```python
from build123d import *
from build123d.topology import SkipClean

# Parameters (mm, degrees)
SKETCH_1_W      = 47
SKETCH_1_H      = 38
SKETCH_1_R      = 1.5
EXTRUDE_1_DEPTH = 3
SKETCH_2_W      = 47
SKETCH_2_H      = 11
SKETCH_2_R      = 1.5
EXTRUDE_2_DEPTH = 7
EXTRUDE_3_DEPTH = 8
FILLET_4_R      = 3
EXTRUDE_4_DEPTH = 10
FILLET_6_R      = 3
EXTRUDE_START   = 3
SKETCH_7_R      = 3.5
SKETCH_7_R_2    = 1.5
EXTRUDE_5_DEPTH = 3


with BuildPart() as part:
    # 草图1 → 凸台-拉伸1 (new body)
    with BuildSketch(Plane(origin=(0, 0, 0), x_dir=(1, 0, 0), z_dir=(0, 1, 0))):
        Rectangle(SKETCH_1_W, SKETCH_1_H)
        with Locations(Location((19.5, 14, 0), (0, 0, 270))):
            Circle(SKETCH_1_R, mode=Mode.SUBTRACT)
        with Locations(Location((19.5, -14, 0), (0, 0, 270))):
            Circle(SKETCH_1_R, mode=Mode.SUBTRACT)
        with Locations(Location((-19.5, -14, 0), (0, 0, 270))):
            Circle(SKETCH_1_R, mode=Mode.SUBTRACT)
        with Locations(Location((-19.5, 14, 0), (0, 0, 270))):
            Circle(SKETCH_1_R, mode=Mode.SUBTRACT)
    extrude(amount=EXTRUDE_1_DEPTH)

    # 草图2 → 凸台-拉伸2 (add)
    with BuildSketch(Plane.XY.offset(19)):
        with Locations((0, 5.5)):
            Rectangle(SKETCH_2_W, SKETCH_2_H)
        with Locations((-17.5, 7)):
            Circle(SKETCH_2_R, mode=Mode.SUBTRACT)
        with Locations((-9.5, 7)):
            Circle(SKETCH_2_R, mode=Mode.SUBTRACT)
    extrude(amount=EXTRUDE_2_DEPTH)

    # 草图3 → 凸台-拉伸3 (add)
    with BuildSketch(Plane(origin=(0, 0, 0), x_dir=(0, 0, -1), z_dir=(1, 0, 0))):
        Polygon((-19, 11), (-19, 8), (-4, 3), (5, 3), align=None)
    extrude(amount=EXTRUDE_3_DEPTH)

    # 圆角4
    fillet_4_edges = [part.edges().sort_by_distance(p)[0] for p in [
        (-23.5, 11, 22.5),
        (23.5, 11, 22.5),
    ]]
    fillet(fillet_4_edges, radius=FILLET_4_R)

    # 草图4 → 凸台-拉伸4 (add)
    with BuildSketch(Plane.ZY.offset(23.5)):
        Polygon((26, 0), (26, -5), (23, -5), (19.5, 0), align=None)
    extrude_4 = extrude(amount=-EXTRUDE_4_DEPTH)

    # 镜向1: 凸台-拉伸4 across plane
    add(extrude_4.mirror(Plane(origin=(0, 0, 0), x_dir=(0, 0, 1), z_dir=(1, 0, 0))))

    # 圆角6
    fillet_6_edges = [part.edges().sort_by_distance(p)[0] for p in [
        (-23.5, 1.5, -19),
        (23.5, 1.5, -19),
    ]]
    fillet(fillet_6_edges, radius=FILLET_6_R)

    # 草图7 → 凸台-拉伸5 (add)
    with SkipClean():  # the faces are left unmerged after this step: merging them gives an invalid solid
        with BuildSketch(Plane(origin=(0, 0, 19), x_dir=(-1, 0, 0), z_dir=(0, 0, -1)).offset(EXTRUDE_START)):
            with Locations(Location((9.5, 7, 0), (0, 0, 180))):
                Circle(SKETCH_7_R)
            with Locations((9.5, 7)):
                Circle(SKETCH_7_R_2, mode=Mode.SUBTRACT)
        extrude(amount=-EXTRUDE_5_DEPTH)


solid = part.part
```
Source: CAD feature listing. Evaluate the final solid. Frame: model axes, mm. A direction names the side the tool comes from. Give positions to 0.01 mm unless a question says otherwise; leave off trailing zeros. Write each loop counter-clockwise with the first axis right and the second up, starting at its lowest first coordinate (ties: lowest second). Pieces come first, ordered by that corner, then holes. Notation, with made-up numbers: (-37.5, 55) - (-15.5, 55) arc R19 cw to (-15.5, 78) - close; hole circle Ø7 at (11.5, 83). An arc over 180 degrees is marked (long way). One line per item, written item: value. Start each with the question number.
Q1. Set-up query: faces 1 (the face through (-13.5, -2, 24)), 2 (the face through (-12.3, 9.1, 17.5)), 3 (the face through (0, 6, 10)). Return all of +Z, -Z, +X, -X, +Y, -Y with unobstructed straight access to the full face (end or side cutting, diameter ignored); none if empty.
Q2. First-contact query: pin 1 Ø13.5 at (x, z) = (-1, 5.5) entering from -Y; pin 2 Ø3.5 at (x, y) = (-9.5, 7) entering from +Z; pin 3 Ø5 at (x, z) = (-19.5, 14) entering from +Y; pin 4 Ø4 at (x, z) = (3.5, 13) entering from +Y. Flat tips, straight axial feed; report the tip coordinate or a pass-through.
Q3. Section query D-D, the plane x = 19.5. Return the cut outline in (y, z), then the cut area to 3 significant figures.
Q4. Material intervals for probe 1 along X at (y, z) = (1.5, -14); probe 2 along Y at (x, z) = (-9, -9.5); probe 3 along Z at (x, y) = (-19, 0.25), sorted ascending. Write a range as from..to.
Q5. Section query A-A, the plane z = -14. Return the cut outline in (x, y), then the cut area to 3 significant figures.
Q6. Draft query along Z for faces 4 (the face through (-19, -5, 25)), 5 (the face through (20.51, 1.48, 12.89)), 6 (the face through (0, 1, -19)). Return one class per face: +Z half, -Z half, draft (parallel to the pull), parting line (faces both ways), or undercut.
Answer:
1. face 1: +Z, -Z, -Y
1. face 2: -Z
1. face 3: -Z, +Y
2. pin 1: stops at y = 0
2. pin 2: stops at z = 26
2. pin 3: stops at y = 3
2. pin 4: stops at y = 9.67
3. outline: (-5, 23) - (0, 19.5) - (0, 15.5) - (3, 15.5) - (3, 19) - (11, 19) - (11, 26) - (-5, 26) - close; (0, -19) - (3, -19) - (3, -15.5) - (0, -15.5) - close; (0, -12.5) - (3, -12.5) - (3, 12.5) - (0, 12.5) - close
3. area: 197 mm2
4. probe 1: x = -23.5..-21, -18..18, 21..23.5
4. probe 2: y = 0..3
4. probe 3: z = -19..-15.41, -12.59..12.59, 15.41..26
5. outline: (-23.5, 0) - (-21, 0) - (-21, 3) - (-23.5, 3) - close; (-18, 0) - (18, 0) - (18, 3) - (-18, 3) - close; (21, 0) - (23.5, 0) - (23.5, 3) - (21, 3) - close
5. area: 123 mm2
6. face 4: draft
6. face 5: undercut
6. face 6: -Z half
